Input: dimensioned drawing with shaded views. Units: mm. Origin: part minimum x, y, z. Round coordinates to 2 decimals unless told otherwise and drop trailing zeros. Loops run counter-clockwise (first coordinate to the right, second up) from the corner with the lowest first, then second, coordinate; pieces in that order, holes last. Notation, with made-up numbers: (-37.75, 60) - (21.25, 60) arc R21 cw to (21.25, 79) - close; hole circle Ø3 at (-38.75, 24.25). An arc over 180 degrees is marked (long way). One line per question, with ' | ' between items.
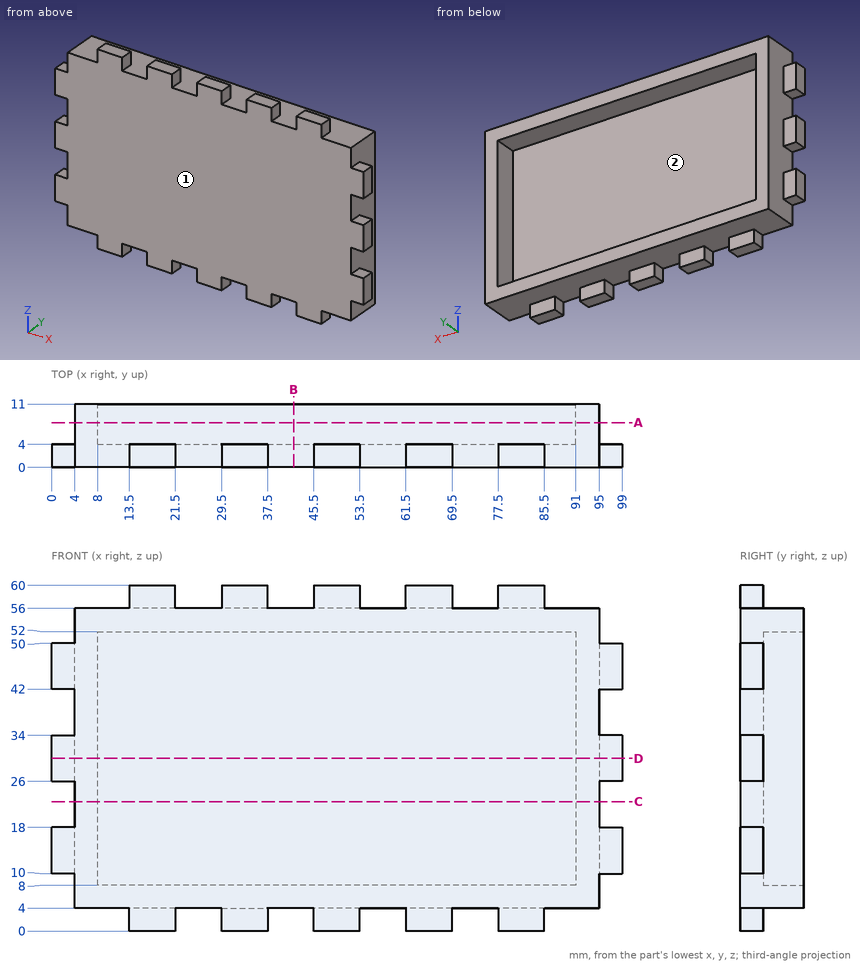
1. Material intervals for probe 1 along Z at (x, y) = (23.5, 8.75); probe 2 along X at (y, z) = (7.5, 44); probe 3 along Y at (x, z) = (41, 30), sorted ascending.
Worked out:
probe 1: z = 4 to 8, 52 to 56 | probe 2: x = 4 to 8, 91 to 95 | probe 3: y = 0 to 4
2. Mould query, pull axis X, two halves, no side actions, for the marked faces 1 and 2. Classes: released by +X, released by -X, zero draft, split by the parting line, or undercut.
Worked out:
face 1: zero draft | face 2: undercut
3. Section query A-A, the plane y = 7.75. Return loops of the section in (x, z), plus the area to 3 significant figures.
Worked out:
outline: (4, 4) - (95, 4) - (95, 56) - (4, 56) - close; hole (8, 8) - (91, 8) - (91, 52) - (8, 52) - close | area: 1,080 mm2
4. Section query C-C, the plane z = 22.5. Return loops of the section in (x, y).
Worked out:
outline: (4, 0) - (95, 0) - (95, 11) - (91, 11) - (91, 4) - (8, 4) - (8, 11) - (4, 11) - close
5. Contact query for flat-ended pins moving along their axis: P1, Ø3.5, axis at y = 6, z = 26, coming from the +X side; P2, Ø4, axis at x = 47.5, y = 8, coming from the +Z side; P3, Ø2, axis at x = 19, z = 59, coming from the +Y side. Output: stop coordinate, or through.
Worked out:
P1: stops at x = 95 | P2: stops at z = 56 | P3: stops at y = 4
6. Section query B-B, the plane x = 42. Return loops of the section in (y, z).
Worked out:
outline: (0, 4) - (11, 4) - (11, 8) - (4, 8) - (4, 52) - (11, 52) - (11, 56) - (0, 56) - close
7. Section query D-D, the plane z = 30. Return loops of the section in (x, y).
Worked out:
outline: (0, 0) - (99, 0) - (99, 4) - (95, 4) - (95, 11) - (91, 11) - (91, 4) - (8, 4) - (8, 11) - (4, 11) - (4, 4) - (0, 4) - close
